```python
from build123d import *

# Parameters (mm, degrees)
BOSS_EXTRUDE1_DEPTH = 9.82
SKETCH3_R           = 1.5
BOSS_EXTRUDE2_DEPTH = 6
SKETCH5_R           = 1
BOSS_EXTRUDE3_DEPTH = 4
FILLET1_R           = 1
FILLET3_R           = 1


with BuildPart() as part:
    # Sketch2 → Boss-Extrude1 (new body)
    with BuildSketch(Plane.XY):
        Polygon((0, 10), (5.6, 10), (5.6, 19), (70.6, 19), (70.6, 10), (76.2, 10), (76.2, 0), (63.1, 0), (63.1, 7.5), (13.1, 7.5), (13.1, 0), (0, 0), align=None)
    extrude(amount=-BOSS_EXTRUDE1_DEPTH)

    # Sketch3 → Boss-Extrude2 (add)
    with BuildSketch(Plane(origin=(0, 19, 0), x_dir=(1, 0, 0), z_dir=(0, 1, 0))):
        with Locations(Location((9.4, 1.5, 0), (0, 0, 270))):
            Circle(SKETCH3_R)
        with Locations(Location((66.8, 1.5, 0), (0, 0, 90))):
            Circle(SKETCH3_R)
    extrude(amount=BOSS_EXTRUDE2_DEPTH)

    # Sketch5 → Boss-Extrude3 (add)
    with BuildSketch(Plane.XZ):
        with Locations(Location((73.025, -8.32, 0), (0, 0, 270))):
            Circle(SKETCH5_R)
        with Locations(Location((3.175, -8.32, 0), (0, 0, 90))):
            Circle(SKETCH5_R)
    extrude(amount=BOSS_EXTRUDE3_DEPTH)

    # Fillet1
    fillet1_edges = [part.edges().sort_by_distance(p)[0] for p in [
        (38.1, 7.5, 0),
    ]]
    fillet(fillet1_edges, radius=FILLET1_R)

    # Fillet3
    # the kernel refuses this fillet: 1 mm, written as the material it adds along each edge
    with BuildSketch(Plane(origin=(63.1, 7.5, -1), x_dir=(-1, 0, 0), z_dir=(0, 0, -1))) as fillet3_piece_1:
        with BuildLine():
            CenterArc((FILLET3_R, -FILLET3_R), FILLET3_R, 90, 90)
            Line((0, -FILLET3_R), (0, 0))
            Line((0, 0), (FILLET3_R, 0))
        make_face()
    extrude(amount=8.82)
    with BuildSketch(Plane(origin=(13.1, 7.5, -1), x_dir=(1, 0, 0), z_dir=(0, 0, -1))) as fillet3_piece_2:
        with BuildLine():
            CenterArc((FILLET3_R, FILLET3_R), FILLET3_R, 180, 90)
            Line((0, FILLET3_R), (0, 0))
            Line((0, 0), (FILLET3_R, 0))
        make_face()
    extrude(amount=8.82)
    with BuildSketch(Plane(origin=(63.1, 8.5, -1), x_dir=(0, 0.5976672776328268, -0.8017442392976488), z_dir=(0, -0.8017442392976488, -0.5976672776328268))) as fillet3_piece_3_section:
        with BuildLine():
            CenterArc((1 + FILLET3_R, -FILLET3_R), FILLET3_R, 90, 90)
            Line((1 + FILLET3_R, 0), (1, 0))
            Line((1, 0), (1, -FILLET3_R))
        make_face()
    fillet3_piece_3 = revolve(axis=Axis((63.1, 8.5, -1), (1, 0, 0)), revolution_arc=233.296989237, mode=Mode.PRIVATE)
    fillet3_piece_3 = split(fillet3_piece_3, bisect_by=Plane(origin=(62.788371694, 7.750061053, 0), z_dir=(0, 0, -1)), keep=Keep.TOP, mode=Mode.PRIVATE)
    add(fillet3_piece_3)
    with BuildSketch(Plane(origin=(13.1, 8.5, -1), x_dir=(0, 0.5976672776328246, -0.8017442392976504), z_dir=(0, -0.8017442392976504, -0.5976672776328246))) as fillet3_piece_4_section:
        with BuildLine():
            CenterArc((1 + FILLET3_R, FILLET3_R), FILLET3_R, 180, 90)
            Line((1, FILLET3_R), (1, 0))
            Line((1, 0), (1 + FILLET3_R, 0))
        make_face()
    fillet3_piece_4 = revolve(axis=Axis((13.1, 8.5, -1), (1, 0, 0)), revolution_arc=233.296989237, mode=Mode.PRIVATE)
    fillet3_piece_4 = split(fillet3_piece_4, bisect_by=Plane(origin=(13.411628296, 7.750061029, 0), z_dir=(0, 0, -1)), keep=Keep.TOP, mode=Mode.PRIVATE)
    add(fillet3_piece_4)
    # the kernel refuses this fillet: 1 mm, written as the material it takes off along each edge
    with BuildSketch(Plane(origin=(63.1, 0, 2.5), x_dir=(0, 1, 0), z_dir=(0, 0, -1)), Plane(origin=(13.1, 0, 2.5), x_dir=(-1, 0, 0), z_dir=(0, 0, -1)), Plane(origin=(0, 10, 2.5), x_dir=(1, 0, 0), z_dir=(0, 0, -1)), Plane(origin=(76.2, 10, 2.5), x_dir=(0, -1, 0), z_dir=(0, 0, -1))) as fillet3_2_piece_1:
        with BuildLine():
            CenterArc((FILLET3_R, FILLET3_R), FILLET3_R, 180, 90)
            Line((0, FILLET3_R), (0, 0))
            Line((0, 0), (FILLET3_R, 0))
        make_face()
    extrude(amount=14.82, mode=Mode.SUBTRACT)


solid = part.part
```
Can you work these out from the model? Positions are in its coordinate system, mm. A direction names the side the tool comes from. Give positions to 0.01 mm unless a question says otherwise; leave off trailing zeros. Order: outer loops, then holes, each group sorted by start corner. A loop starts at its lowest first (then second) coordinate and runs counter-clockwise, first axis right, second up. Notation, with made-up numbers: (51.25, 25) - (87.25, 25) arc R29 ccw to (87.25, 61) - close; hole circle Ø7 at (-6.75, -30). An arc over 180 degrees is marked (long way). Use a Markdown table: item, result. Add a question column.
Q1. If we mould it in two halves opening along X, with no side actions, what happens to faces 6 (the flat face through (63.1, 4, -5)), 7 (the flat face through (38, 7.5, -5)), 8 (the flat face through (9, 25, -2)), 9 (the flat face through (0, 4, -5))? For each: released by +X, released by -X, zero draft, split by the parting line, or undercut.
Q2. On a 3-axis mill with a long thin cutter (end or side, diameter ignored), from which of +Z, -Z, +X, -X, +Y, -Y can I reach the whole of each face in a straight line? I mean faces 1 (the cylindrical face through (2.875, -1.972, -7.366)), 2 (the flat face through (73, 10, -5)), 3 (the flat face through (5.6, 14, -5)), 4 (the cylindrical face through (10.887, 21.958, -1.695)), 5 (the flat face through (13.1, 4, -5)). Say none if no direction works.
Q3. If we section it at D-D on y = 23: Write out the boundary of the cut face in (x, z).
Q4. If we section it at C-C on x = 24: Write out the boundary of the cut face in (y, z), plus the area to 3 significant figures.
Q5. I'm going to push flat-ended pins straight in: pin 1 (3.5 mm diameter, centred on x = 72.5, z = -2.5, fed in from +Y); pin 2 (5 mm diameter, centred on x = 68, z = -3, fed in from -Y); pin 3 (1 mm diameter, centred on x = 29.5, z = -8, fed in from -Y). Where does each tip first touch, or does it pass through?
Q6. If we section it at B-B on z = -5.75: Write out the boundary of the cut face in (x, y), plus the area to 3 significant figures.
Q7. Please list where these lines run through material, in increasing order: line 1 along X through (y, z) = (2.75, -9); line 2 along X through (y, z) = (-0.5, -8.5); line 3 along X through (y, z) = (13.5, -6.25).
Q8. If we section it at A-A on y = 3.75: Write out the boundary of the cut face in (x, z), plus the area to 3 significant figures.
Answers follow:
| question | item | result |
|---|---|---|
| 1 | face 6 | undercut |
| 1 | face 7 | undercut |
| 1 | face 8 | zero draft |
| 1 | face 9 | released by -X |
| 2 | face 1 | -Y |
| 2 | face 2 | +Z, -Z, +X, +Y |
| 2 | face 3 | +Z, -Z, -X, +Y |
| 2 | face 4 | +Y |
| 2 | face 5 | +Z, -Z, -Y |
| 3 | outline | circle Ø3 at (9.4, -1.5); circle Ø3 at (66.8, -1.5) |
| 4 | outline | (7.5, -9.82) - (19, -9.82) - (19, 0) - (8.5, 0) arc R1 ccw to (7.5, -1) - close |
| 4 | area | 113 mm^2 |
| 5 | pin 1 | stops at y = 10 |
| 5 | pin 2 | stops at y = 0 |
| 5 | pin 3 | stops at y = 7.5 |
| 6 | outline | (0, 0) - (12.1, 0) arc R1 ccw to (13.1, 1) - (13.1, 6.5) arc R1 cw to (14.1, 7.5) - (62.1, 7.5) arc R1 cw to (63.1, 6.5) - (63.1, 1) arc R1 ccw to (64.1, 0) - (76.2, 0) - (76.2, 9) arc R1 ccw to (75.2, 10) - (70.6, 10) - (70.6, 19) - (5.6, 19) - (5.6, 10) - (1, 10) arc R1 ccw to (0, 9) - close |
| 6 | area | 972 mm^2 |
| 7 | line 1 | x = 0 to 13.1, 63.1 to 76.2 |
| 7 | line 2 | x = 2.19 to 4.16, 72.04 to 74.01 |
| 7 | line 3 | x = 5.6 to 70.6 |
| 8 | outline | (0, -9.82) - (13.1, -9.82) - (13.1, 0) - (0, 0) - close; (63.1, -9.82) - (76.2, -9.82) - (76.2, 0) - (63.1, 0) - close |
| 8 | area | 257 mm^2 |
